from build123d import *

# Parameters (mm, degrees)
CROQUIS1_W              = 9.8
CROQUIS1_H              = 9.8
SALIENTE_EXTRUIR1_DEPTH = 22
REDONDEO1_R             = 1
CROQUIS2_R              = 1.5
CORTAR_EXTRUIR1_DEPTH   = 7
CROQUIS3_R              = 2
CORTAR_EXTRUIR2_DEPTH   = 5.2


with BuildPart() as part:
    # Croquis1 → Saliente-Extruir1 (new body)
    with BuildSketch(Plane.XY):
        with Locations((-4.9, 4.9)):
            Rectangle(CROQUIS1_W, CROQUIS1_H)
    extrude(amount=SALIENTE_EXTRUIR1_DEPTH)

    # Redondeo1
    redondeo1_edges = [part.edges().sort_by_distance(p)[0] for p in [
        (0, 4.9, 22),
        (-4.9, 9.8, 0),
        (0, 4.9, 0),
        (0, 9.8, 11),
        (-4.9, 9.8, 22),
    ]]
    fillet(redondeo1_edges, radius=REDONDEO1_R)

    # Croquis2 → Cortar-Extruir1 (cut)
    with BuildSketch(Plane.ZY.offset(9.8)):
        with Locations((11, 4.4)):
            Circle(CROQUIS2_R)
    extrude(amount=-CORTAR_EXTRUIR1_DEPTH, mode=Mode.SUBTRACT)

    # Croquis3 → Cortar-Extruir2 (cut)
    with BuildSketch(Plane.XZ):
        with Locations((-5.4, 18.5)):
            Circle(CROQUIS3_R)
        with Locations((-5.4, 3.5)):
            Circle(CROQUIS3_R)
    extrude(amount=-CORTAR_EXTRUIR2_DEPTH, mode=Mode.SUBTRACT)


solid = part.part
For this review, take the finished solid that the model builds, in its own axes (mm). A direction names the side the tool comes from. Give positions to 0.01 mm unless a question says otherwise; leave off trailing zeros. Loops run counter-clockwise (first coordinate to the right, second up) from the corner with the lowest first, then second, coordinate; pieces in that order, holes last. Notation, with made-up numbers: M 36,69 L 61,69 A36 cw 61,104 Z; hole C 76,-17 d1. An arc over 180 degrees is marked long. Answer as a JSON object with one key per item and string values. Group by question number.
Q1. For probe 1 along Z at (x, y) = (-5.4, 1.95); probe 2 along Z at (x, y) = (-5.4, 3.2); probe 3 along Z at (x, y) = (-4.5, 1.75), list the stretches that pass through material, from the lowest coordinate up. Write a range as [from, to].
Q2. Add section A-A on y = 4.4. Give the boundary of the cut face in (x, z).
Q3. Add section B-B on x = -5.4. Give the boundary of the cut face in (y, z), and give its area (3 significant figures).
Q4. Mouldability with a two-part tool opening along X and no side actions: class faces 1 (the flat face through (-5, 5.2, 19)), 2 (the flat face through (-5, 4, 22)), 3 (the cylindrical face through (-0.285, 4.462, 21.699)) as +X half, -X half, draft (parallel to the pull), parting line (faces both ways), or undercut.
Q5. Add section D-D on z = 3.5. Give the boundary of the cut face in (x, y), and give its area (3 significant figures).
Q6. Tool access review of faces 4 (the flat face through (-2.8, 4, 11)), 5 (the cylindrical face through (-5.338, 9.515, 21.699)), 6 (the cylindrical face through (-5.66, 2.564, 20.483)): name each direction out of +Z, -Z, +X, -X, +Y, -Y from which nothing blocks a thin tool from reaching the whole face with its end or side.
Q7. Add section C-C on z = 11. Give the boundary of the cut face in (x, y).
Q8. Insertion check: P1, Ø2, axis at x = -6, z = 3.5, coming from the -Y side; P2, Ø1.5, axis at y = 4, z = 11.5, coming from the -X side. Each pin has a flat end and moves straight along its axis. Give the tip position at first contact, or say it passes through.
Checked values:
{
 "1": {"probe 1": "[0, 1.5], [5.5, 16.5], [20.5, 22]", "probe 2": "[0, 1.5], [5.5, 10.1], [11.9, 16.5], [20.5, 22]", "probe 3": "[0, 1.71], [5.29, 16.71], [20.29, 22]"},
 "2": {"outline": "M -9.8,0 L -1,0 A1 ccw 0,1 L 0,21 A1 ccw -1,22 L -9.8,22 L -9.8,12.5 L -2.8,12.5 L -2.8,9.5 L -9.8,9.5 Z; hole C -5.4,3.5 d4; hole C -5.4,18.5 d4"},
 "3": {"outline": "M 0,0 L 8.8,0 A1 ccw 9.8,1 L 9.8,21 A1 ccw 8.8,22 L 0,22 L 0,20.5 L 5.2,20.5 L 5.2,16.5 L 0,16.5 L 0,5.5 L 5.2,5.5 L 5.2,1.5 L 0,1.5 Z; hole C 4.4,11 d3", "area": "167 mm²"},
 "4": {"face 1": "undercut", "face 2": "draft", "face 3": "+X half"},
 "5": {"outline": "M -9.8,0 L -7.4,0 L -7.4,5.2 L -3.4,5.2 L -3.4,0 L 0,0 L 0,8.8 A1 ccw -1,9.8 L -9.8,9.8 Z", "area": "75.0 mm²"},
 "6": {"face 4": "-X", "face 5": "+Z, +X, -X, +Y", "face 6": "-Y"},
 "7": {"outline": "M -9.8,0 L 0,0 L 0,8.8 A1 ccw -1,9.8 L -9.8,9.8 L -9.8,5.9 L -2.8,5.9 L -2.8,2.9 L -9.8,2.9 Z"},
 "8": {"P1": "y = 5.2", "P2": "x = -2.8"}
}
